Design review of the part built by this model. Coordinates are the model's own, in mm. A direction names the side the tool comes from. Coordinates: 2 decimals unless noted, no trailing zeros. Loops run counter-clockwise (first coordinate to the right, second up) from the corner with the lowest first, then second, coordinate; pieces in that order, holes last. Notation, with made-up numbers: (4.25, -33) -> (11.25, -33) arc R22 ccw to (11.25, -23) -> close; hole circle Ø7 at (9, 75). An arc over 180 degrees is marked (long way). Answer as a JSON object with one key per item and string values.
Autodesk Inventor part; units mm, degrees
ref_plane "YZ Plane" through (0, 0, 0) normal (1, 0, 0) x (0, 1, 0)
ref_plane "XZ Plane" through (0, 0, 0) normal (0, 1, 0) x (-1, 0, 0)
ref_plane "XY Plane" through (0, 0, 0) normal (0, 0, 1) x (1, 0, 0)
sketch "Sketch1" plane through (0, 0, 0) normal (1, 0, 0) x (0, 1, 0)
  line L0 (-15, 15) -> (15, 15)
  line L1 (15, 15) -> (15, -15)
  line L2 (15, -15) -> (-15, -15)
  line L3 (-15, -15) -> (-15, 15)
  line L4 (-15, 15) -> (15, -15) construction
  line L5 (15, 15) -> (-15, -15) construction
  point P0 (0, 0)
  dimension "d0" = 30
  dimension "d1" = 30
extrude "Extrusion1" add sketch "Sketch1" along normal blind 3
sketch "Sketch2" plane through (0, 0, 0) normal (1, 0, 0) x (0, 1, 0)
  circle A0 centre (0, 0) radius 12.7
  dimension "d4" = 25.4
extrude "Extrusion2" cut sketch "Sketch2" along normal blind 1.614
sketch "Sketch3" plane through (0, 0, 0) normal (-1, 0, 0) x (0, 0, 1)
  circle A0 centre (0, 0) radius 12
  dimension "d7" = 24
extrude "Extrusion3" cut sketch "Sketch3" against normal up to next
sketch "Sketch4" plane through (0, 0, 0) normal (0, 1, 0) x (-1, 0, 0)
  line L0 (-1.614, 12.7) -> (-1.614, -12.7)
  line L1 (-1.614, 0) -> (-1.614, -12.5586)
  line L2 (-2.2305, 0) -> (-1.614, 0)
  arc A0 (-2.2305, 0) -> (-1.614, -12.5586) centre (125.9995, 0) ccw
  point P0 (0, 0)
  dimension "d10" = 12.5586
  dimension "d11" = 256.46
revolve "Revolution1" cut sketch "Sketch4" angle 360 about axis through (2.2305, 0, 0) along (-1, 0, 0)
sketch "Sketch7" plane through (3, 0, 0) normal (1, 0, 0) x (0, 0, -1)
  circle A0 centre (12, 12) radius 1.5
  circle A1 centre (12, -12) radius 1.5
  circle A2 centre (-9, -12) radius 1.5
  line L0 (15, 15) -> (-15, 15)
  line L1 (15, -15) -> (15, 15)
  line L2 (-15, -15) -> (15, -15)
  line L3 (-15, 15) -> (-15, -15)
  point P0 (0, 0)
  dimension "d24" = 3
  dimension "d25" = 3
  dimension "d26" = 3
  dimension "d27" = 3
  dimension "d28" = 3
  dimension "d29" = 3
  dimension "d30" = 6
extrude "Extrusion6" cut sketch "Sketch7" against normal up to surface (3 mm away) contours A0 | A1 | A2
sketch "Sketch8" plane through (3, 0, 0) normal (1, 0, 0) x (0, 0, -1)
  line L0 (0, 0) -> (-15, 0) construction
  line L1 (-15, 15) -> (-15, -15)
  line L2 (0, 0) -> (-11.75, -8.2274)
  line L3 (-11.75, -8.2274) -> (-11.75, -15)
  line L4 (-15, -15) -> (15, -15)
  line L5 (-11.75, -15) -> (-15, -15)
  line L6 (-15, -15) -> (-15, 0)
  line L7 (-15, -15) -> (-15, 15)
  line L8 (0, 0) -> (-11.75, 8.2274)
  line L9 (-11.75, 8.2274) -> (-11.75, 15)
  line L10 (-15, 15) -> (15, 15)
  dimension "d33" = 3.25
  dimension "d34" = 35
extrude "Extrusion7" cut sketch "Sketch8" against normal up to surface (3 mm away)
properties part number "LargeLensHolderP2S1" material "Acetal Resin, Black"
1) For faces 4 (the flat face through (1.5, -7.7, 11)), 5 (the cylindrical face through (1.52, -11.93, 10.5)), 6 (the cylindrical face through (0.796, 0.45, -12.692)), list the 3-axis set-ups (+Z, -Z, +X, -X, +Y, -Y) from which the entire face can be reached by the end or side of a thin tool; tool diameter is ignored.
Completed:
{"face 4": "+Z, +X, -X", "face 5": "+X, -X", "face 6": "-X"}
2) Wall thickness on probe 1 along Z at (x, y) = (1.7, -12.75); probe 2 along Y at (x, z) = (1, 9); probe 3 along Y at (x, z) = (0.9, 0): over which ranges is each line inside the solid? List them lowest first.
Completed:
{"probe 1": "-15 to -13.3, -10.7 to 7.7, 10.3 to 11.75", "probe 2": "-15 to -13.5, -10.5 to -8.96, 8.96 to 15", "probe 3": "-15 to -12.7, 12.7 to 15"}
3) Add section A-A, the plane x = 2.1. Give the boundary of the cut face in (y, z).
Completed:
{"outline": "(-15, -15) -> (15, -15) -> (15, 11.75) -> (8.23, 11.75) -> (6.88, 9.83) arc R12 cw (long way) to (-6.88, 9.83) -> (-8.23, 11.75) -> (-15, 11.75) -> close; hole circle Ø3 at (-12, -12); hole circle Ø3 at (-12, 9); hole circle Ø3 at (12, -12)"}
4) The part is to be moulded in two halves that separate along Z. For faces 1 (the flat face through (1, 15, -1)), 2 (the flat face through (1.5, 7.7, 11)), 3 (the cylindrical face through (2, 0, -12)), say which applies: pulls with the +Z half, pulls with the -Z half, needs draft (parallel to the pull), parting line crosses it, or undercut.
Completed:
{"face 1": "needs draft", "face 2": "pulls with the +Z half", "face 3": "undercut"}
5) Clearance check with flat-ended pins moving along their axes: pin 1 Ø4 at (y, z) = (-5.5, -11) entering from -X; pin 2 Ø1.5 at (x, y) = (1, -5) entering from +Z. State where each tip first meets the part, or that it passes through.
Completed:
{"pin 1": "x = 0", "pin 2": "z = -10.75"}
6) Add section B-B, the plane z = -11. Count the separate pieces of the cut face and the enclosed holes in it, and give its area (3 significant figures).
Completed:
{"separate pieces": "4", "enclosed holes": "0", "area": "42.7 mm²"}
